The listing builds one solid part. Answer for the finished solid, in the listing's coordinates (mm). A direction names the side the tool comes from. Give positions to 0.01 mm unless a question says otherwise; leave off trailing zeros. Order: outer loops, then holes, each group sorted by start corner. A loop starts at its lowest first (then second) coordinate and runs counter-clockwise, first axis right, second up. Notation, with made-up numbers: (21.25, 50.5) - (28.25, 50.5) arc R24 ccw to (28.25, 87.5) - close; hole circle Ø4 at (66, 47). An arc over 180 degrees is marked (long way). Write each question's results on one line, items separated by ' | '. Start each with the question number.
1. Find the intervals of material crossed by L1, parallel to Z at x = 27, y = 9.5; L2, parallel to Y at x = -28, z = 34; L3, parallel to Y at x = -28.5, z = -17.5, in increasing order.
2. Section C-C (x = 6.5) is taken. Give the vertices of the cut face in (y, z), and give its area (3 significant figures).
3. Section D-D (z = 3) is taken. Give the vertices of the cut face in (x, y), and give its area (3 significant figures).
4. Which of the six approach directions +Z, -Z, +X, -X, +Y, -Y give full straight-line access (tool end or side, diameter ignored) to faces 5 (the face through (-28, -6, 6)), 6 (the face through (27.07, -3.976, -27.021)), 7 (the face through (-28, 6, -6))?
5. Section B-B (y = 13.5) is taken. Give the vertices of the cut face in (x, z).
6. Determine the mould class of faces 1 (the face through (-37.773, -0.229, 0.504)), 2 (the face through (28, -6, 6)), 3 (the face through (-29.97, -4, -27.02)), 4 (the face through (28.5, 8.4, -25.5)) for opening direction Y: released by +Y, released by -Y, zero draft, split by the parting line, or undercut.
7. Flat-ended cylindrical pins translate along their axes: pin 1 (2 mm diameter, centred on y = 0, z = 24, fed in from -X); pin 2 (1.5 mm diameter, centred on y = -6.5, z = -26.5, fed in from +X); pin 3 (1.5 mm diameter, centred on y = 12.5, z = 11.5, fed in from -X). Find the tip coordinate at first contact, or state that the pin passes through.
8. Section A-A (z = -31) is taken. Give the vertices of the cut face in (x, y).
from build123d import *

# Parameters (mm, degrees)
PAD_DEPTH                                = 36
SKETCH001_R                              = 1.7
POCKET_DEPTH                             = 30
POCKET001_DEPTH                          = 1.5
POCKET001_MIRRORED_2_DEPTH               = 1.5
SKETCH001_MIRRORED_2_R                   = 1.7
POCKET_MIRRORED_2_DEPTH                  = 30
POCKET001_MIRRORED001_2_DEPTH            = 1.5
SKETCH001_MIRRORED001_2_R                = 1.7
POCKET_MIRRORED001_2_DEPTH               = 30
POCKET001_MIRRORED_2_MIRRORED001_2_DEPTH = 1.5
SKETCH001_MIRRORED_2_MIRRORED001_2_R     = 1.7
POCKET_MIRRORED_2_MIRRORED001_2_DEPTH    = 30


with BuildPart() as part:
    # Sketch → Pad (new body, symmetric)
    with BuildSketch(Plane.XY):
        with BuildLine():
            ThreePointArc((39.5, -16.244608), (0, -5), (-39.5, -16.244608))
            ThreePointArc((-39.5, -16.244608), (-37.772173, 0), (-39.5, 16.244608))
            ThreePointArc((-39.5, 16.244608), (0, 5), (39.5, 16.244608))
            ThreePointArc((39.5, 16.244608), (37.772173, 0), (39.5, -16.244608))
        make_face()
    extrude(amount=PAD_DEPTH, both=True)

    # Sketch001 (on Face6 of Pad) → Pocket (cut)
    with BuildSketch(Plane.XY.offset(36)):
        with Locations((28.5, -6.5)):
            Circle(SKETCH001_R)
    pocket = extrude(amount=-POCKET_DEPTH, mode=Mode.SUBTRACT)

    # Sketch002 (on DatumPlane) → Pocket001 (cut, symmetric)
    with BuildSketch(Plane.XY.offset(27)):
        Polygon((28.5, -3.15), (25.598815, -4.825), (25.598815, -14.825), (31.401185, -14.825), (31.401185, -4.825), align=None)
    pocket001 = extrude(amount=POCKET001_DEPTH, both=True, mode=Mode.SUBTRACT)

    # Sketch002 Mirrored 2 → Pocket001 Mirrored 2 (cut, symmetric)
    with BuildSketch(Plane(origin=(0, 0, 27), x_dir=(1, 0, 0), z_dir=(0, 0, -1))):
        Polygon((28.5, -3.15), (25.598815, -4.825), (25.598815, -14.825), (31.401185, -14.825), (31.401185, -4.825), align=None)
    pocket001_mirrored_2 = extrude(amount=-POCKET001_MIRRORED_2_DEPTH, both=True, mode=Mode.SUBTRACT)

    # Sketch001 Mirrored 2 → Pocket Mirrored 2 (cut)
    with BuildSketch(Plane(origin=(0, 0, 36), x_dir=(1, 0, 0), z_dir=(0, 0, -1))):
        with Locations((28.5, -6.5)):
            Circle(SKETCH001_MIRRORED_2_R)
    pocket_mirrored_2 = extrude(amount=POCKET_MIRRORED_2_DEPTH, mode=Mode.SUBTRACT)

    # Sketch002 Mirrored001 2 → Pocket001 Mirrored001 2 (cut, symmetric)
    with BuildSketch(Plane(origin=(0, 0, 27), x_dir=(-1, 0, 0), z_dir=(0, 0, -1))):
        Polygon((28.5, -3.15), (25.598815, -4.825), (25.598815, -14.825), (31.401185, -14.825), (31.401185, -4.825), align=None)
    pocket001_mirrored001_2 = extrude(amount=-POCKET001_MIRRORED001_2_DEPTH, both=True, mode=Mode.SUBTRACT)

    # Sketch001 Mirrored001 2 → Pocket Mirrored001 2 (cut)
    with BuildSketch(Plane(origin=(0, 0, 36), x_dir=(-1, 0, 0), z_dir=(0, 0, -1))):
        with Locations((28.5, -6.5)):
            Circle(SKETCH001_MIRRORED001_2_R)
    pocket_mirrored001_2 = extrude(amount=POCKET_MIRRORED001_2_DEPTH, mode=Mode.SUBTRACT)

    # Sketch002 Mirrored 2 Mirrored001 2 → Pocket001 Mirrored 2 Mirrored001 2 (cut, symmetric)
    with BuildSketch(Plane(origin=(0, 0, 27), x_dir=(-1, 0, 0), z_dir=(0, 0, 1))):
        Polygon((28.5, -3.15), (25.598815, -4.825), (25.598815, -14.825), (31.401185, -14.825), (31.401185, -4.825), align=None)
    pocket001_mirrored_2_mirrored001_2 = extrude(amount=POCKET001_MIRRORED_2_MIRRORED001_2_DEPTH, both=True, mode=Mode.SUBTRACT)

    # Sketch001 Mirrored 2 Mirrored001 2 → Pocket Mirrored 2 Mirrored001 2 (cut)
    with BuildSketch(Plane(origin=(0, 0, 36), x_dir=(-1, 0, 0), z_dir=(0, 0, 1))):
        with Locations((28.5, -6.5)):
            Circle(SKETCH001_MIRRORED_2_MIRRORED001_2_R)
    pocket_mirrored_2_mirrored001_2 = extrude(amount=-POCKET_MIRRORED_2_MIRRORED001_2_DEPTH, mode=Mode.SUBTRACT)

    # Mirrored002: Pocket001, Pocket, Pocket001 Mirrored 2, Pocket Mirrored 2, Pocket001 Mirrored001 2, Pocket Mirrored001 2, Pocket001 Mirrored 2 Mirrored001 2, Pocket Mirrored 2 Mirrored001 2 across XY
    add(pocket001.mirror(Plane.XY), mode=Mode.SUBTRACT)
    add(pocket.mirror(Plane.XY), mode=Mode.SUBTRACT)
    add(pocket001_mirrored_2.mirror(Plane.XY), mode=Mode.SUBTRACT)
    add(pocket_mirrored_2.mirror(Plane.XY), mode=Mode.SUBTRACT)
    add(pocket001_mirrored001_2.mirror(Plane.XY), mode=Mode.SUBTRACT)
    add(pocket_mirrored001_2.mirror(Plane.XY), mode=Mode.SUBTRACT)
    add(pocket001_mirrored_2_mirrored001_2.mirror(Plane.XY), mode=Mode.SUBTRACT)
    add(pocket_mirrored_2_mirrored001_2.mirror(Plane.XY), mode=Mode.SUBTRACT)


solid = part.part
Reported:
1) L1: -36 to -28.5, -25.5 to 25.5, 28.5 to 36 | L2: -10.42 to -8.12, -4.88 to 4.88, 8.12 to 10.42 | L3: -10.63 to -8.2, -4.8 to 4.8, 8.2 to 10.63
2) outline: (-5.28, -36) - (5.28, -36) - (5.28, 36) - (-5.28, 36) - close | area: 761 mm²
3) outline: (-39.5, -16.24) arc R75 cw to (39.5, -16.24) arc R77.23 cw to (39.5, 16.24) arc R75 cw to (-39.5, 16.24) arc R77.23 cw to start | area: 1,290 mm²
4) face 5: +Z | face 6: -Y | face 7: -Z
5) outline: (-38.96, -36) - (-34.68, -36) - (-34.68, 36) - (-38.96, 36) - close; (34.68, -36) - (38.96, -36) - (38.96, 36) - (34.68, 36) - close
6) face 1: undercut | face 2: undercut | face 3: released by -Y | face 4: zero draft
7) pin 1: x = -37.78 | pin 2: x = 38.11 | pin 3: x = -38.92
8) outline: (-39.5, -16.24) arc R75 cw to (39.5, -16.24) arc R77.23 cw to (39.5, 16.24) arc R75 cw to (-39.5, 16.24) arc R77.23 cw to start; hole circle Ø3.4 at (-28.5, -6.5); hole circle Ø3.4 at (-28.5, 6.5); hole circle Ø3.4 at (28.5, -6.5); hole circle Ø3.4 at (28.5, 6.5)
